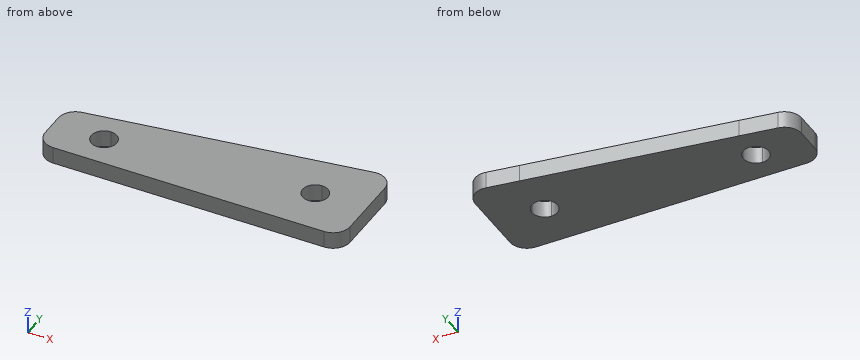
```python
from build123d import *

# Parameters (mm, degrees)
BOSS_EXTRUDE1_DEPTH = 3.175


with BuildPart() as part:
    # Sketch1 → Boss-Extrude1 (new body)
    with BuildSketch(Plane.XY):
        with BuildLine():
            Line((-342.9, 12.065), (-349.720980938, 11.041852859))
            ThreePointArc((-349.720980938, 11.041852859), (-351.655825168, 9.97384631), (-352.425, 7.901979939))
            Line((-352.425, 7.901979939), (-352.425, 3.175))
            ThreePointArc((-352.425, 3.175), (-351.49506403, 0.92993597), (-349.25, 0))
            Line((-349.25, 0), (-342.9, 0))
            Line((-342.9, 0), (-342.9, 3.65125))
            ThreePointArc((-342.9, 3.65125), (-345.28125, 6.0325), (-342.9, 8.41375))
            Line((-342.9, 8.41375), (-342.9, 12.065))
        make_face()
        with BuildLine():
            Line((-304.8, 17.78), (-342.9, 12.065))
            Line((-342.9, 12.065), (-342.9, 8.41375))
            ThreePointArc((-342.9, 8.41375), (-341.216201977, 7.716298023), (-340.51875, 6.0325))
            ThreePointArc((-340.51875, 6.0325), (-341.216201977, 4.348701977), (-342.9, 3.65125))
            Line((-342.9, 3.65125), (-342.9, 0))
            Line((-342.9, 0), (-304.8, 0))
            Line((-304.8, 0), (-304.8, 6.50875))
            ThreePointArc((-304.8, 6.50875), (-307.18125, 8.89), (-304.8, 11.27125))
            Line((-304.8, 11.27125), (-304.8, 17.78))
        make_face()
        with BuildLine():
            Line((-298.920980938, 18.661852859), (-304.8, 17.78))
            Line((-304.8, 17.78), (-304.8, 11.27125))
            ThreePointArc((-304.8, 11.27125), (-303.116201977, 10.573798023), (-302.41875, 8.89))
            ThreePointArc((-302.41875, 8.89), (-303.116201977, 7.206201977), (-304.8, 6.50875))
            Line((-304.8, 6.50875), (-304.8, 0))
            Line((-304.8, 0), (-298.45, 0))
            ThreePointArc((-298.45, 0), (-296.20493597, 0.92993597), (-295.275, 3.175))
            Line((-295.275, 3.175), (-295.275, 15.521979939))
            ThreePointArc((-295.275, 15.521979939), (-296.378133629, 17.927805107), (-298.920980938, 18.661852859))
        make_face()
    extrude(amount=BOSS_EXTRUDE1_DEPTH)


solid = part.part
```
Check sheet for the modelled part. Datum: model origin and axes. Units: mm. Round coordinates to 2 decimals unless told otherwise and drop trailing zeros. Loops run counter-clockwise (first coordinate to the right, second up) from the corner with the lowest first, then second, coordinate; pieces in that order, holes last. Notation, with made-up numbers: M 48,69 L 58,69 A31 ccw 58,101 Z; hole C 39.25,20.25 d6. An arc over 180 degrees is marked long. Answer as a JSON object with one key per item and string values.
1. Section check D-D (y = 14). Record the boundary of the cut face in (x, z) (3 decimals), plus the area to 3 significant figures.
Reply:
{"outline": "M -330,0 L -295.275,0 L -295.275,3.175 L -330,3.175 Z", "area": "110 mm²"}
2. Scan lines: line 1 (Y direction, x = -341, z = 1.45); line 2 (X direction, y = 8.5, z = 1.4) (3 decimals); line 3 (Y direction, x = -304.5, z = 3) (3 decimals). Record each from-to range of solid material in increasing order.
Reply:
{"line 1": "y = 0 to 4.6, 7.47 to 12.35", "line 2": "x = -352.368 to -307.149, -302.451 to -295.275", "line 3": "y = 0 to 6.528, 11.252 to 17.825"}
3. Section check B-B (y = 10.5). Record the boundary of the cut face in (x, z) (1 decimal), plus the area to 3 significant figures.
Reply:
{"outline": "M -351.1,0 L -306.6,0 L -306.6,3.2 L -351.1,3.2 Z; M -303,0 L -295.3,0 L -295.3,3.2 L -303,3.2 Z", "area": "166 mm²"}
4. Section check C-C (x = -338). Record the boundary of the cut face in (y, z) (3 decimals).
Reply:
{"outline": "M 0,0 L 12.8,0 L 12.8,3.175 L 0,3.175 Z"}
5. Section check A-A (z = 0.7). State how many separate pieces and enclosed holes the cut face has, plus the area to 3 significant figures.
Reply:
{"separate pieces": "1", "enclosed holes": "2", "area": "808 mm²"}
